Verification items for the finished model (mm, model axes). A direction names the side the tool comes from. Round coordinates to 2 decimals unless told otherwise and drop trailing zeros. Loops run counter-clockwise (first coordinate to the right, second up) from the corner with the lowest first, then second, coordinate; pieces in that order, holes last. Notation, with made-up numbers: (-23.5, 26.5) - (-14.5, 26.5) arc R22 ccw to (-14.5, 50.5) - close; hole circle Ø4 at (-32, 2.25). An arc over 180 degrees is marked (long way). Use a Markdown table: item, result. Add a question column.
```python
from build123d import *

# Parameters (mm, degrees)
SKIZZE1_W                        = 520
SKIZZE1_H                        = 320
SKIZZE1_W_2                      = 500
SKIZZE1_H_2                      = 300
AUFSATZ_LINEAR_AUSTRAGEN1_DEPTH  = 2
SKIZZE2_W                        = 504
SKIZZE2_H                        = 304
SKIZZE2_W_2                      = 500
SKIZZE2_H_2                      = 300
AUFSATZ_LINEAR_AUSTRAGEN2_DEPTH  = 15
AUFSATZ_LINEAR_AUSTRAGEN3_DEPTH  = 280
AUFSATZ_LINEAR_AUSTRAGEN4_REACH  = 654.656
SKIZZE4_W                        = 2
SKIZZE4_H                        = 20
AUFSATZ_LINEAR_AUSTRAGEN5_REACH  = 662.576
SKIZZE5_W                        = 2
SKIZZE5_H                        = 20
AUFSATZ_LINEAR_AUSTRAGEN7_DEPTH  = 2
AUFSATZ_LINEAR_AUSTRAGEN12_DEPTH = 254
AUFSATZ_LINEAR_AUSTRAGEN13_DEPTH = 254
AUFSATZ_LINEAR_AUSTRAGEN16_DEPTH = 504
AUFSATZ_LINEAR_AUSTRAGEN17_REACH = 737.316
SKIZZE12_W                       = 20
SKIZZE12_H                       = 2
AUFSATZ_LINEAR_AUSTRAGEN18_REACH = 624.098
SKIZZE13_W                       = 20
SKIZZE13_H                       = 2


with BuildPart() as part:
    # Skizze1 → Aufsatz-Linear austragen1 (new body)
    with BuildSketch(Plane(origin=(0, 0, 0), x_dir=(1, 0, 0), z_dir=(0, 1, 0))):
        with Locations((260, 160)):
            Rectangle(SKIZZE1_W, SKIZZE1_H)
        with Locations((260, 160)):
            Rectangle(SKIZZE1_W_2, SKIZZE1_H_2, mode=Mode.SUBTRACT)
    extrude(amount=AUFSATZ_LINEAR_AUSTRAGEN1_DEPTH)

    # Skizze2 → Aufsatz-Linear austragen2 (add)
    with BuildSketch(Plane(origin=(0, 2, 0), x_dir=(1, 0, 0), z_dir=(0, 1, 0))):
        with Locations((260, 160)):
            Rectangle(SKIZZE2_W, SKIZZE2_H)
        with Locations((260, 160)):
            Rectangle(SKIZZE2_W_2, SKIZZE2_H_2, mode=Mode.SUBTRACT)
    extrude(amount=AUFSATZ_LINEAR_AUSTRAGEN2_DEPTH)

    # Skizze3 → Aufsatz-Linear austragen3 (add)
    with BuildSketch(Plane(origin=(0, 2, 0), x_dir=(1, 0, 0), z_dir=(0, 1, 0))):
        Polygon((8, 294), (6, 294), (6, 314), (26, 314), (26, 312), (8, 312), align=None)
        Polygon((512, 312), (512, 294), (514, 294), (514, 314), (494, 314), (494, 312), align=None)
        Polygon((512, 26), (514, 26), (514, 6), (494, 6), (494, 8), (512, 8), align=None)
        Polygon((8, 8), (8, 26), (6, 26), (6, 6), (26, 6), (26, 8), align=None)
    extrude(amount=AUFSATZ_LINEAR_AUSTRAGEN3_DEPTH)

    # Skizze4 → Aufsatz-Linear austragen4 (add, up to next)
    with BuildSketch(Plane(origin=(26, 0, 0), x_dir=(0, 0, -1), z_dir=(1, 0, 0)), mode=Mode.PRIVATE) as aufsatz_linear_austragen4_sk1:
        with Locations((7, 272)):
            Rectangle(SKIZZE4_W, SKIZZE4_H)
    aufsatz_linear_austragen4_tool1 = extrude(aufsatz_linear_austragen4_sk1.sketch, amount=AUFSATZ_LINEAR_AUSTRAGEN4_REACH, mode=Mode.PRIVATE) - part.part
    aufsatz_linear_austragen4 = aufsatz_linear_austragen4_tool1.solids().sort_by_distance((26, 272, -7))[0]
    add(aufsatz_linear_austragen4)

    # Spiegeln1: Aufsatz-Linear austragen4 across plane
    add(aufsatz_linear_austragen4.mirror(Plane.XY.offset(-160)))

    # Skizze5 → Aufsatz-Linear austragen5 (add, up to next)
    with BuildSketch(Plane.XY.offset(-294), mode=Mode.PRIVATE) as aufsatz_linear_austragen5_sk1:
        with Locations((513, 272)):
            Rectangle(SKIZZE5_W, SKIZZE5_H)
    aufsatz_linear_austragen5_tool1 = extrude(aufsatz_linear_austragen5_sk1.sketch, amount=AUFSATZ_LINEAR_AUSTRAGEN5_REACH, mode=Mode.PRIVATE) - part.part
    aufsatz_linear_austragen5 = aufsatz_linear_austragen5_tool1.solids().sort_by_distance((513, 272, -294))[0]
    add(aufsatz_linear_austragen5)

    # Spiegeln2: Aufsatz-Linear austragen5 across plane
    add(aufsatz_linear_austragen5.mirror(Plane(origin=(260, 0, 0), x_dir=(0, 0, 1), z_dir=(1, 0, 0))))

    # Skizze7 → Aufsatz-Linear austragen7 (add)
    with BuildSketch(Plane.ZY.offset(-6)):
        Polygon((-314, 282), (-160, 393.283421946), (-6, 282), (-40.147044848, 282), (-160, 368.608097271), (-279.852955152, 282), align=None)
    aufsatz_linear_austragen7 = extrude(amount=-AUFSATZ_LINEAR_AUSTRAGEN7_DEPTH)

    # Spiegeln5: Aufsatz-Linear austragen7 across plane
    add(aufsatz_linear_austragen7.mirror(Plane(origin=(260, 0, 0), x_dir=(0, 0, 1), z_dir=(1, 0, 0))))

    # Skizze8 → Aufsatz-Linear austragen12 (add)
    with BuildSketch(Plane(origin=(260, 0, 0), x_dir=(0, 0, -1), z_dir=(1, 0, 0))):
        Polygon((175.039121874, 382.415857367), (160, 393.283421946), (144.960878126, 382.415857367), (143.789473684, 384.036909998), (160, 395.750954413), (176.210526316, 384.036909998), align=None)
    extrude(amount=AUFSATZ_LINEAR_AUSTRAGEN12_DEPTH)

    # Skizze8<2> → Aufsatz-Linear austragen13 (add)
    with BuildSketch(Plane(origin=(260, 0, 0), x_dir=(0, 0, -1), z_dir=(1, 0, 0))):
        Polygon((175.039121874, 382.415857367), (160, 393.283421946), (144.960878126, 382.415857367), (143.789473684, 384.036909998), (160, 395.750954413), (176.210526316, 384.036909998), align=None)
    extrude(amount=-AUFSATZ_LINEAR_AUSTRAGEN13_DEPTH)

    # Skizze11 → Aufsatz-Linear austragen16 (add)
    with BuildSketch(Plane.ZY.offset(-512)):
        Polygon((-314, 282), (-312, 282), (-312, 280), (-310.585295515, 280), (-310.585295515, 282), (-296.618069243, 292.092991784), (-297.789473684, 293.714044415), align=None)
    aufsatz_linear_austragen16 = extrude(amount=AUFSATZ_LINEAR_AUSTRAGEN16_DEPTH)

    # Spiegeln6: Aufsatz-Linear austragen16 across plane
    add(aufsatz_linear_austragen16.mirror(Plane.XY.offset(-160)))

    # Aufsatz-Linear austragen17: up to this plane
    aufsatz_linear_austragen17_end = Plane(origin=(6, 282, -314), z_dir=(0, 0, 1))
    # Skizze12 → Aufsatz-Linear austragen17 (add, up to the surface)
    with BuildSketch(Plane(origin=(0, 48.090839316, 66.550696637), x_dir=(-1, 0, 0), z_dir=(0, -0.5857022207681483, -0.8105263157894748)), mode=Mode.PRIVATE) as aufsatz_linear_austragen17_sk1:
        with Locations((-16, 413.478918374)):
            Rectangle(SKIZZE12_W, SKIZZE12_H)
    aufsatz_linear_austragen17_tool1 = split(extrude(aufsatz_linear_austragen17_sk1.sketch, amount=AUFSATZ_LINEAR_AUSTRAGEN17_REACH, mode=Mode.PRIVATE), bisect_by=aufsatz_linear_austragen17_end, keep=Keep.BOTH, mode=Mode.PRIVATE)
    aufsatz_linear_austragen17 = aufsatz_linear_austragen17_tool1.solids().sort_by_distance((16, 383.226384, -175.624824))[0]
    add(aufsatz_linear_austragen17)

    # Spiegeln10: Aufsatz-Linear austragen17 across plane
    add(aufsatz_linear_austragen17.mirror(Plane(origin=(260, 0, 0), x_dir=(0, 0, 1), z_dir=(1, 0, 0))))

    # Aufsatz-Linear austragen18: up to this plane
    aufsatz_linear_austragen18_end = Plane(origin=(514, 282, -6), z_dir=(0, 0, -1))
    # Skizze13 → Aufsatz-Linear austragen18 (add, up to the surface)
    with BuildSketch(Plane(origin=(0, 200.003499524, -276.775627385), x_dir=(1, 0, 0), z_dir=(0, -0.5857022207681525, 0.8105263157894717)), mode=Mode.PRIVATE) as aufsatz_linear_austragen18_sk1:
        with Locations((16, 226.054207728)):
            Rectangle(SKIZZE13_W, SKIZZE13_H)
    aufsatz_linear_austragen18_tool1 = split(extrude(aufsatz_linear_austragen18_sk1.sketch, amount=AUFSATZ_LINEAR_AUSTRAGEN18_REACH, mode=Mode.PRIVATE), bisect_by=aufsatz_linear_austragen18_end, keep=Keep.BOTH, mode=Mode.PRIVATE)
    aufsatz_linear_austragen18 = aufsatz_linear_austragen18_tool1.solids().sort_by_distance((16, 383.226384, -144.375176))[0]
    add(aufsatz_linear_austragen18)

    # Spiegeln12: Aufsatz-Linear austragen18 across plane
    add(aufsatz_linear_austragen18.mirror(Plane(origin=(260, 0, 0), x_dir=(0, 0, 1), z_dir=(1, 0, 0))))


solid = part.part
```
Q1. Thickness scan on line 1 along X through (y, z) = (303.5, -256.5); line 2 along Y through (x, z) = (369.5, -307). Record the ranges inside material, lowest first.
Q2. Section check C-C on y = 143.5. Record the cut outline in (x, z), plus the area to 3 significant figures.
Q3. Section check B-B on y = 268. Record the cut outline in (x, z), plus the area to 3 significant figures.
Q4. Set-up check for faces 1 (the face through (280, 269, -314)), 2 (the face through (510, 8, -158)), 3 (the face through (512, 276, -159)), 4 (the face through (6, 265, -149)), 5 (the face through (257, 9, -312)): record each of +Z, -Z, +X, -X, +Y, -Y from which the full face is reachable in a straight line by a thin tool's end or side.
Q5. Go/stop test with flat-tipped pins: pin 1 Ø1.6 at (x, z) = (513, -109.5) entering from +Y; pin 2 Ø13.5 at (x, y) = (333.5, 10) entering from +Z; pin 3 Ø2 at (x, y) = (513.5, 129.5) entering from -Z. Record where each tip stops, or that it passes through.
Q6. Section check A-A on x = 373.5. State how many separate pieces and enclosed holes the cut face has, plus the area to 3 significant figures.
Q7. Release check for a two-part mould opening along Z. For faces 6 (the face through (259, 265, -8)), 7 (the face through (513.014, 324.698, -99.235)), 8 (the face through (257, 9, -8)), 9 (the face through (182, 0, -315)) record: +Z half, -Z half, draft (parallel to the pull), parting line (faces both ways), or undercut.
Determined:
| question | item | result |
|---|---|---|
| 1 | line 1 | x = 6 to 8, 512 to 514 |
| 1 | line 2 | y = 284.59 to 287.06 |
| 2 | outline | (6, -314) - (26, -314) - (26, -312) - (8, -312) - (8, -294) - (6, -294) - close; (6, -26) - (8, -26) - (8, -8) - (26, -8) - (26, -6) - (6, -6) - close; (494, -314) - (514, -314) - (514, -294) - (512, -294) - (512, -312) - (494, -312) - close; (494, -8) - (512, -8) - (512, -26) - (514, -26) - (514, -6) - (494, -6) - close |
| 2 | area | 304 mm² |
| 3 | outline | (6, -314) - (514, -314) - (514, -6) - (6, -6) - close; hole (8, -312) - (512, -312) - (512, -8) - (8, -8) - close |
| 3 | area | 3,250 mm² |
| 4 | face 1 | -Z, +X, -X, +Y |
| 4 | face 2 | -Y |
| 4 | face 3 | none |
| 4 | face 4 | +Z, -Z, -X, +Y |
| 4 | face 5 | -Z |
| 5 | pin 1 | stops at y = 359.84 |
| 5 | pin 2 | stops at z = -8 |
| 5 | pin 3 | stops at z = -314 |
| 6 | separate pieces | 5 |
| 6 | enclosed holes | 0 |
| 6 | area | 337 mm² |
| 7 | face 6 | undercut |
| 7 | face 7 | undercut |
| 7 | face 8 | +Z half |
| 7 | face 9 | draft |
